```python
from build123d import *

# Parameters (mm, degrees)
F0_W     = 177.8
F0_H     = 304.8
F1_DEPTH = 6.35
F3_DEPTH = 25.4


with BuildPart() as f1:
    # F0 (on Front) → F1 (new body)
    with BuildSketch(Plane.XZ):
        Rectangle(F0_W, F0_H)
    extrude(amount=F1_DEPTH)

    # F2 (on face) → F3 (cut)
    with BuildSketch(Plane.XZ.offset(6.35)):
        with BuildLine():
            Line((50.8, 152.4), (-50.8, 152.4))
            ThreePointArc((-50.8, 152.4), (0, 101.6), (50.8, 152.4))
        make_face()
    extrude(amount=-F3_DEPTH, mode=Mode.SUBTRACT)


solid = f1.part
```
Design review of the part built by this model. Coordinates are the model's own, in mm. Give positions to 0.01 mm unless a question says otherwise; leave off trailing zeros. Write each loop counter-clockwise with the first axis right and the second up, starting at its lowest first coordinate (ties: lowest second). Pieces come first, ordered by that corner, then holes. Notation, with made-up numbers: (23, -37) -> (72, -37) arc R24 cw to (72, -23) -> close; hole circle Ø11 at (56, -14.75). An arc over 180 degrees is marked (long way). Answer in a Markdown table with one row per item.
(1) Mouldability with a two-part tool opening along X and no side actions: class faces 1 (the cylindrical face through (-1.117, -3.219, 101.612)), 2 (the flat face through (88.9, -3, -2)), 3 (the flat face through (-1, -6.35, 2)) as +X half, -X half, draft (parallel to the pull), parting line (faces both ways), or undercut.
Results:
| item | result |
|---|---|
| face 1 | undercut |
| face 2 | +X half |
| face 3 | draft |
(2) Consider section D-D (x = -45.5). State the section outline as (y, z) points.
Results:
| item | result |
|---|---|
| outline | (-6.35, -152.4) -> (0, -152.4) -> (0, 129.81) -> (-6.35, 129.81) -> close |
(3) Consider section B-B (x = 0). State the section outline as (y, z) points.
Results:
| item | result |
|---|---|
| outline | (-6.35, -152.4) -> (0, -152.4) -> (0, 101.6) -> (-6.35, 101.6) -> close |
(4) Consider section A-A (z = 132). State the section outline as (x, y) points, then the cut area to 3 significant figures.
Results:
| item | result |
|---|---|
| outline | (-88.9, -6.35) -> (-46.52, -6.35) -> (-46.52, 0) -> (-88.9, 0) -> close; (46.52, -6.35) -> (88.9, -6.35) -> (88.9, 0) -> (46.52, 0) -> close |
| area | 538 mm2 |
(5) To check wall thickness, follow probe 1 along Z at (x, y) = (-2, -1.75); probe 2 along Z at (x, y) = (-36.5, -2.5); probe 3 along X at (y, z) = (-3.25, 132). State the ranges of each line that lie inside material, in increasing order.
Results:
| item | result |
|---|---|
| probe 1 | -152.4 to 101.64 |
| probe 2 | -152.4 to 117.07 |
| probe 3 | -88.9 to -46.52, 46.52 to 88.9 |
(6) Consider section C-C (y = -4.5). State the section outline as (x, z) points.
Results:
| item | result |
|---|---|
| outline | (-88.9, -152.4) -> (88.9, -152.4) -> (88.9, 152.4) -> (50.8, 152.4) arc R50.8 cw to (-50.8, 152.4) -> (-88.9, 152.4) -> close |
